```python
from build123d import *

# Parameters (mm, degrees)
SKETCH6_R                = 13.75
SKETCH6_R_2              = 11
BOSS_EXTRUDE2_DEPTH      = 7
SKETCH4_W                = 5.4
SKETCH4_H                = 1.75
BOSS_EXTRUDE3_REACH      = 30.322
SKETCH9_W                = 7
SKETCH9_H                = 9.16515139
BOSS_EXTRUDE4_START      = 0.75
SKETCH10_R               = 13.75
SKETCH10_R_2             = 13
BOSS_EXTRUDE4_DEPTH      = 0.75
CHAMFER1_SIZE            = 0.5
CHAMFER1_OF_MIRROR1_SIZE = 0.5
BOSS_EXTRUDE5_DEPTH      = 1.55
BOSS_EXTRUDE5_START      = 5.45
BOSS_EXTRUDE5_2_DEPTH    = 1.55
FILLET1_R                = 2
SKETCH12_W               = 1.554666846
SKETCH12_H               = 4.45309529
SKETCH12_W_2             = 1.373791393
SKETCH12_H_2             = 2.545281327
SKETCH12_W_3             = 0.712647602
SKETCH12_H_3             = 1.069707629
SKETCH12_W_4             = 1.072015963
SKETCH12_W_5             = 0.597408117
SKETCH12_H_4             = 1.399070537
SKETCH12_W_6             = 0.336309622
CUT_EXTRUDE1_DEPTH       = 1
SKETCH14_R               = 11
CUT_EXTRUDE2_DEPTH       = 21.667002685


# Read off the part's stored shape, not the designer's step: Boss-Extrude5
with BuildPart() as part:
    # Sketch6 → Boss-Extrude2 (new body)
    with BuildSketch(Plane(origin=(0, 0, 0), x_dir=(0, 0, -1), z_dir=(1, 0, 0))):
        Circle(SKETCH6_R)
        Circle(SKETCH6_R_2, mode=Mode.SUBTRACT)
    extrude(amount=BOSS_EXTRUDE2_DEPTH)

    # Sketch4 → Cut-Revolve1 (revolve, cut)
    with BuildSketch(Plane.XY, mode=Mode.PRIVATE) as cut_revolve1_sk:
        with Locations((3.5, -12.875)):
            Rectangle(SKETCH4_W, SKETCH4_H)
    revolve(cut_revolve1_sk.sketch.rotate(Axis((-11.602577702, 0, 0), (1, 0, 0)), 270), axis=Axis((-11.602577702, 0, 0), (1, 0, 0)), mode=Mode.SUBTRACT)

    # Sketch9 → Boss-Extrude3 (add, up to next)
    with BuildSketch(Plane.XY.offset(-10), mode=Mode.PRIVATE) as boss_extrude3_sk1:
        with Locations((3.5, 0)):
            Rectangle(SKETCH9_W, SKETCH9_H)
    boss_extrude3_tool1 = extrude(boss_extrude3_sk1.sketch, amount=-BOSS_EXTRUDE3_REACH, mode=Mode.PRIVATE) - part.part
    add(boss_extrude3_tool1.solids().sort_by_distance((3.5, 0, -10))[0])

    # Sketch10 → Boss-Extrude4 (add)
    with BuildSketch(Plane.ZY.offset(-6.2).offset(BOSS_EXTRUDE4_START)):
        Circle(SKETCH10_R)
        Circle(SKETCH10_R_2, mode=Mode.SUBTRACT)
    boss_extrude4 = extrude(amount=-BOSS_EXTRUDE4_DEPTH)

    # Chamfer1
    chamfer1_edges = [part.edges().sort_by_distance(p)[0] for p in [
        (5.45, 0, -13),
    ]]
    chamfer(chamfer1_edges, length=CHAMFER1_SIZE)

    # Mirror1: Boss-Extrude4 across plane
    add(boss_extrude4.mirror(Plane.ZY.offset(-3.5)))

    # Chamfer1 of Mirror1
    chamfer1_of_mirror1_edges = [part.edges().sort_by_distance(p)[0] for p in [
        (1.55, 0, -13),
    ]]
    chamfer(chamfer1_of_mirror1_edges, length=CHAMFER1_OF_MIRROR1_SIZE)

    # Boss-Extrude5 outline → Boss-Extrude5 (add)
    with BuildSketch(Plane.YZ):
        with BuildLine():
            ThreePointArc((0, -13.75), (-2.917586852, -13.436896478), (-5.7023, -12.511845376))
            Line((-5.7023, -12.511845376), (-5.7023, -13.75))
            Line((-5.7023, -13.75), (0, -13.75))
        make_face()
        with BuildLine():
            ThreePointArc((5.7023, -12.511845376), (2.917586852, -13.436896478), (0, -13.75))
            Line((0, -13.75), (5.7023, -13.75))
            Line((5.7023, -13.75), (5.7023, -12.511845376))
        make_face()
    extrude(amount=BOSS_EXTRUDE5_DEPTH)

    # Boss-Extrude5 2 outline → Boss-Extrude5 2 (add)
    with BuildSketch(Plane.YZ.offset(BOSS_EXTRUDE5_START)):
        with BuildLine():
            ThreePointArc((0, -13.75), (-2.917586852, -13.436896478), (-5.7023, -12.511845376))
            Line((-5.7023, -12.511845376), (-5.7023, -13.75))
            Line((-5.7023, -13.75), (0, -13.75))
        make_face()
        with BuildLine():
            ThreePointArc((5.7023, -12.511845376), (2.917586852, -13.436896478), (0, -13.75))
            Line((0, -13.75), (5.7023, -13.75))
            Line((5.7023, -13.75), (5.7023, -12.511845376))
        make_face()
    extrude(amount=BOSS_EXTRUDE5_2_DEPTH)

    # Fillet1
    fillet1_edges = [part.edges().sort_by_distance(p)[0] for p in [
        (6.225, -5.7023, -12.511845376),
        (6.225, 5.7023, -12.511845376),
        (0.775, -5.7023, -12.511845376),
        (0.775, 5.7023, -12.511845376),
    ]]
    fillet(fillet1_edges, radius=FILLET1_R)

    # Sketch12 → Cut-Extrude1 (cut)
    with BuildSketch(Plane(origin=(0, 0, -13.75), x_dir=(-1, 0, 0), z_dir=(0, 0, -1))):
        with Locations((-5.370167958, -3.135823217)):
            Rectangle(SKETCH12_W, SKETCH12_H)
        Polygon((-4.592834535, -0.909275572), (-4.592834535, -1.672246677), (-3.997102403, -1.672246677), (-3.997102403, -0.27317614), (-5.19036655, -0.27317614), (-5.19036655, -0.909275572), align=None)
        with Locations((-5.279730232, 1.561396449)):
            Rectangle(SKETCH12_W_2, SKETCH12_H_2)
        with Locations((-1.906323801, 0.675050165)):
            Rectangle(SKETCH12_W_3, SKETCH12_H_3)
        with Locations((-1.013992018, 0.675050165)):
            Rectangle(SKETCH12_W_4, SKETCH12_H_3)
        with Locations((-1.848704059, -0.972711409)):
            Rectangle(SKETCH12_W_5, SKETCH12_H_4)
        with Locations((-1.381845189, -0.972711409)):
            Rectangle(SKETCH12_W_6, SKETCH12_H_4)
    extrude(amount=-CUT_EXTRUDE1_DEPTH, mode=Mode.SUBTRACT)

    # Sketch14 → Cut-Extrude2 (cut, through all)
    with BuildSketch(Plane(origin=(7, 0, 0), x_dir=(0, 0, -1), z_dir=(1, 0, 0))):
        Circle(SKETCH14_R)
    extrude(amount=-CUT_EXTRUDE2_DEPTH, mode=Mode.SUBTRACT)


solid = part.part
```
Work out the finished part from the listing and answer in its coordinate system (mm). A direction names the side the tool comes from. Coordinates: 2 decimals unless noted, no trailing zeros. Order: outer loops, then holes, each group sorted by start corner. A loop starts at its lowest first (then second) coordinate and runs counter-clockwise, first axis right, second up. Notation, with made-up numbers: M 5,48.5 L 46,48.5 A32 ccw 46,74.5 Z; hole C 43.5,66 d3. An arc over 180 degrees is marked long. Use CSV: the item, a comma, the result in double quotes.
1) Consider line 1 (Y direction, x = 0.9, z = 0); line 2 (X direction, y = 12.25, z = -0.75); line 3 (Y direction, x = 1.5, z = 0). Determine where each line is inside the solid, lowest interval first. Write a range as [from, to].
Worked out:
line 1,"y = [-13.75, -13], [-12, -11], [11, 12], [13, 13.75]"
line 2,"x = [0, 0.8], [6.2, 7]"
line 3,"y = [-13.75, -13.45], [-12, -11], [11, 12], [13.45, 13.75]"
2) For faces 4 (the face through (6.148, -3, -13)), 5 (the face through (5.815, -0.541, 13.124)), 6 (the face through (6.21, -5.97, -12.74)), determine the directions among +Z, -Z, +X, -X, +Y, -Y from which every point of the face is accessible in a straight line to the end or side of a thin tool.
Worked out:
face 4,"-Z"
face 5,"none"
face 6,"-Z, +X, -X, -Y"
3) Section A-A on z = 0 is taken. Write down the section's boundary in (x, y).
Worked out:
outline,"M 0,-13.75 L 1.55,-13.75 L 1.55,-13.5 L 1.05,-13 L 0.8,-13 L 0.8,-12 L 6.2,-12 L 6.2,-13 L 5.95,-13 L 5.45,-13.5 L 5.45,-13.75 L 7,-13.75 L 7,-11 L 0,-11 Z; M 0,11 L 7,11 L 7,13.75 L 5.45,13.75 L 5.45,13.5 L 5.95,13 L 6.2,13 L 6.2,12 L 0.8,12 L 0.8,13 L 1.05,13 L 1.55,13.5 L 1.55,13.75 L 0,13.75 Z"
4) Flat-ended cylindrical pins translate along their axes: pin 1 Ø4 at (x, y) = (2, 8) entering from +Z; pin 2 Ø0.8 at (x, z) = (5.5, -13.5) entering from -Y; pin 3 Ø1.1 at (x, z) = (1, -13) entering from -Y. Find the tip coordinate at first contact, or state that the pin passes through.
Worked out:
pin 1,"stops at z = 12.35"
pin 2,"stops at y = -5.81"
pin 3,"stops at y = -6.17"
5) Determine the mould class of faces 1 (the face through (0.478, 1, -13)), 2 (the face through (6.2, 9, 9)), 3 (the face through (0.79, -0.51, 13.74)) for opening direction Z: released by +Z, released by -Z, zero draft, split by the parting line, or undercut.
Worked out:
face 1,"zero draft"
face 2,"undercut"
face 3,"split by the parting line"
6) Section B-B on x = 3.75 is taken. Write down the section's boundary in (y, z), plus the area to 3 significant figures.
Worked out:
outline,"C 0,0 d24; hole C 0,0 d22"
area,"72.3 mm^2"
